Geometry check sheet. Reference: the model listing, model coordinates, mm. A direction names the side the tool comes from. Give positions to 0.01 mm unless a question says otherwise; leave off trailing zeros. Loops run counter-clockwise (first coordinate to the right, second up) from the corner with the lowest first, then second, coordinate; pieces in that order, holes last. Notation, with made-up numbers: (57.5, 24) -> (66.5, 24) arc R24 ccw to (66.5, 35) -> close; hole circle Ø3 at (27.5, 56.5). An arc over 180 degrees is marked (long way). One line per item, written item: value. Start each with the question number.
(1) Sectioned sample at A-A, the plane y = -19. Record the cut outline in (x, z), then the cut area to 3 significant figures.
(2) Scan lines: line 1 along Z through (x, y) = (137, 126); line 2 along Y through (x, z) = (139.5, 17.5). Record each from-to range of solid material in increasing order. Write a range as from..to.
(3) Sectioned sample at B-B, the plane x = 138. Record the cut outline in (y, z).
(4) Tool access check on faces 4 (the face through (-142, 176.281, 14)), 5 (the face through (3, 53, 0)). Record the directions out of +Z, -Z, +X, -X, +Y, -Y that give a thin tool (end or side, any length) a straight path to the whole face; none if there is none.
(5) Sectioned sample at C-C, the plane x = 0. Record the cut outline in (y, z), then the cut area to 3 significant figures.
(6) Draft check along X on faces 1 (the face through (-135, 177.8, 10)), 2 (the face through (-166.613, 177.051, 13.37)), 3 (the face through (-179.319, 50.2, 0.4)). Enter one of: pulls with the +X half, pulls with the -X half, needs draft (parallel to the pull), parting line crosses it, or undercut.
from build123d import *

# Parameters (mm, degrees)
BOTTOM_CENTER_CASING_DEPTH = 1.51892
SKETCH3_W                  = 76.2
SKETCH3_H                  = 1.51892
BOSS_EXTRUDE1_DEPTH        = 25.4
SKETCH4_R                  = 6.35
CUT_EXTRUDE1_DEPTH         = 25.4


with BuildPart() as part:
    # Sketch1 → Bottom Center Casing (new body)
    with BuildSketch(Plane.XY):
        with BuildLine():
            Line((-179.31892, 177.8), (-15, 177.8))
            ThreePointArc((-15, 177.8), (0, 162.8), (15, 177.8))
            Line((15, 177.8), (179.31892, 177.8))
            Line((179.31892, 177.8), (179.31892, -76.2))
            Line((179.31892, -76.2), (-179.31892, -76.2))
            Line((-179.31892, -76.2), (-179.31892, 177.8))
        make_face()
    extrude(amount=BOTTOM_CENTER_CASING_DEPTH)

    # Sketch3 → Boss-Extrude1 (add)
    with BuildSketch(Plane.XY.offset(1.51892)):
        with Locations((-141.21892, 177.04054)):
            Rectangle(SKETCH3_W, SKETCH3_H)
        with Locations((141.21892, 177.04054)):
            Rectangle(SKETCH3_W, SKETCH3_H)
    extrude(amount=BOSS_EXTRUDE1_DEPTH)

    # Sketch4 → Cut-Extrude1 (cut)
    with BuildSketch(Plane(origin=(0, 177.8, 0), x_dir=(1, 0, 0), z_dir=(0, 1, 0))):
        with Locations((-160.26892, -13.649325)):
            Circle(SKETCH4_R)
        with Locations((-122.16892, -14.029055)):
            Circle(SKETCH4_R)
        with Locations((122.16892, -14.029055)):
            Circle(SKETCH4_R)
        with Locations((160.26892, -13.649325)):
            Circle(SKETCH4_R)
    extrude(amount=-CUT_EXTRUDE1_DEPTH, mode=Mode.SUBTRACT)


solid = part.part
Calculated:
1. outline: (-179.32, 0) -> (179.32, 0) -> (179.32, 1.52) -> (-179.32, 1.52) -> close
1. area: 545 mm2
2. line 1: z = 0..1.52
2. line 2: y = 176.28..177.8
3. outline: (-76.2, 0) -> (177.8, 0) -> (177.8, 26.92) -> (176.28, 26.92) -> (176.28, 1.52) -> (-76.2, 1.52) -> close
4. face 4: +Z, +X, -X, -Y
4. face 5: -Z, +X, -X, +Y, -Y
5. outline: (-76.2, 0) -> (162.8, 0) -> (162.8, 1.52) -> (-76.2, 1.52) -> close
5. area: 363 mm2
6. face 1: needs draft
6. face 2: undercut
6. face 3: pulls with the -X half
